Read the model definition and answer for the solid it produces. Units are mm, in the model's axes. A direction names the side the tool comes from. Give positions to 0.01 mm unless a question says otherwise; leave off trailing zeros. Order: outer loops, then holes, each group sorted by start corner. A loop starts at its lowest first (then second) coordinate and runs counter-clockwise, first axis right, second up.
```python
from build123d import *

# Parameters (mm, degrees)
EXTRUDE_THIN1_DEPTH = 70
SKETCH2_W           = 40
SKETCH2_H           = 8
CUT_EXTRUDE1_DEPTH  = 10
SKETCH3_W           = 20
SKETCH3_H           = 100
CUT_EXTRUDE2_DEPTH  = 90
SKETCH9_R           = 20
CUT_EXTRUDE9_DEPTH  = 2


with BuildPart() as part:
    # Sketch1 → Extrude-Thin1 (new body)
    with BuildSketch(Plane(origin=(0, 0, 0), x_dir=(0, 0, -1), z_dir=(1, 0, 0))):
        with BuildLine():
            Line((-38.022129, 0), (58.945617271, 0))
            ThreePointArc((58.945617271, 0), (66.879150674, 3.91238571), (68.604875534, 12.588190451))
            Line((68.604875534, 12.588190451), (34.909714379, 138.34024385))
            ThreePointArc((34.909714379, 138.34024385), (30.732716209, 142.003372931), (25.749958229, 139.546148624))
            Line((25.749958229, 139.546148624), (-30.714507865, 41.746824527))
            ThreePointArc((-30.714507865, 41.746824527), (-33.750539659, 39.417195395), (-37.544634884, 39.916697508))
            Line((-37.544634884, 39.916697508), (-46.204888922, 44.916697508))
            Line((-46.204888922, 44.916697508), (-45.204888922, 46.648748316))
            Line((-45.204888922, 46.648748316), (-36.544634884, 41.648748316))
            ThreePointArc((-36.544634884, 41.648748316), (-34.268177749, 41.349047048), (-32.446558673, 42.746824527))
            Line((-32.446558673, 42.746824527), (24.017907421, 140.546148624))
            ThreePointArc((24.017907421, 140.546148624), (30.993768593, 143.986262654), (36.841566032, 138.85788194))
            Line((36.841566032, 138.85788194), (70.536727187, 13.105828541))
            ThreePointArc((70.536727187, 13.105828541), (68.465857355, 2.694862852), (58.945617271, -2))
            Line((58.945617271, -2), (-38.022129, -2))
            Line((-38.022129, -2), (-38.022129, 0))
        make_face()
    extrude(amount=EXTRUDE_THIN1_DEPTH)

    # Sketch2 → Cut-Extrude1 (cut)
    with BuildSketch(Plane(origin=(0, 15.412270146, -8.898278318), x_dir=(1, 0, 0), z_dir=(0, 0.8660254037844438, -0.4999999999999912))):
        with Locations((35, -58.472956339)):
            Rectangle(SKETCH2_W, SKETCH2_H)
    extrude(amount=-CUT_EXTRUDE1_DEPTH, mode=Mode.SUBTRACT)

    # Sketch3 → Cut-Extrude2 (cut)
    with BuildSketch(Plane.XY):
        with Locations((35, 12.152835355)):
            Rectangle(SKETCH3_W, SKETCH3_H)
    extrude(amount=-CUT_EXTRUDE2_DEPTH, mode=Mode.SUBTRACT)

    # Sketch9 → Cut-Extrude9 (cut)
    with BuildSketch(Plane(origin=(0, 24.73647817, 42.84483699), x_dir=(1, 0, 0), z_dir=(0, 0.4999999999999915, 0.8660254037844435))):
        with Locations(Location((35, 77.261022729, 0), (0, 0, 270))):
            Circle(SKETCH9_R)
    extrude(amount=-CUT_EXTRUDE9_DEPTH, mode=Mode.SUBTRACT)


solid = part.part
```
1) The part is cut by section D-D on y = 59.5. Determine the outline of the cut face in (x, z).
Final values:
outline: (0, -58.11) - (25, -58.11) - (25, -56.03) - (0, -56.03) - close; (0, 20.46) - (70, 20.46) - (70, 22.77) - (0, 22.77) - close; (45, -58.11) - (70, -58.11) - (70, -56.03) - (45, -56.03) - close
2) Given pin 1 (3 mm diameter, centred on x = 39.5, y = 123.5, fed in from -Z); pin 2 (4 mm diameter, centred on x = 55, y = 93, fed in from +Z); pin 3 (1 mm diameter, centred on x = 39, y = -1, fed in from -Z), each flat-ended and moving along its own axis, determine where each tip first touches the part or whether it passes through.
Final values:
pin 1: stops at z = -41.36
pin 2: stops at z = 4.59
pin 3: stops at z = 0
3) For a pull along Y with two mould halves and no side action, classify faces 1 (the face through (18.95, 102.2, -4.19)), 2 (the face through (34.51, 76.862, -53.453)), 3 (the face through (45, -1, -48)) as released by +Y, released by -Y, zero draft, split by the parting line, or undercut.
Final values:
face 1: undercut
face 2: released by +Y
face 3: zero draft
4) A tool of negligible diameter and unlimited length cuts with its end or side. For faces 4 (the face through (34.51, 42.52, 38.05)), 5 (the face through (35, 0, 1)), 6 (the face through (34.51, 141.992, -30.814)), 7 (the face through (25, -1, -48)), 8 (the face through (54.83, 93.41, 2.06)), from which of +Z, -Z, +X, -X, +Y, -Y can it reach the whole face along a straight path? Write none if from no direction.
Final values:
face 4: +X, -X, +Y
face 5: +Z, +X, -X
face 6: +X, -X
face 7: -Z, -Y
face 8: none
5) Consider L1, parallel to Y at x = 56.5, z = 26; L2, parallel to Z at x = 36.5, y = 119.5; L3, parallel to Z at x = 22, y = 70. Determine where each line is inside the solid, lowest interval first.
Final values:
L1: y = -2 to 0, 49.91 to 53.91
L2: z = -42.03 to -39.96, -14.18 to -11.87
L3: z = -55.29 to -53.22, 14.4 to 16.71
6) The part is cut by section A-A on z = 22. Determine the outline of the cut face in (x, y).
Final values:
outline: (0, -2) - (70, -2) - (70, 0) - (0, 0) - close; (0, 56.84) - (70, 56.84) - (70, 60.84) - (0, 60.84) - close
7) The part is cut by section B-B on y = 22.5. Determine the outline of the cut face in (x, z), and give its area (3 significant figures).
Final values:
outline: (0, -68.02) - (25, -68.02) - (25, -65.95) - (0, -65.95) - close; (45, -68.02) - (70, -68.02) - (70, -65.95) - (45, -65.95) - close
area: 104 mm2
8) The part is cut by section C-C on x = 9. Determine the outline of the cut face in (y, z).
Final values:
outline: (-2, -58.95) arc R12 ccw to (13.11, -70.54) - (138.86, -36.84) arc R7 ccw to (140.55, -24.02) - (42.75, 32.45) arc R3 cw to (41.65, 36.54) - (46.65, 45.2) - (44.92, 46.2) - (39.92, 37.54) arc R5 ccw to (41.75, 30.71) - (139.55, -25.75) arc R5 cw to (138.34, -34.91) - (12.59, -68.6) arc R10 cw to (0, -58.95) - (0, 38.02) - (-2, 38.02) - close
